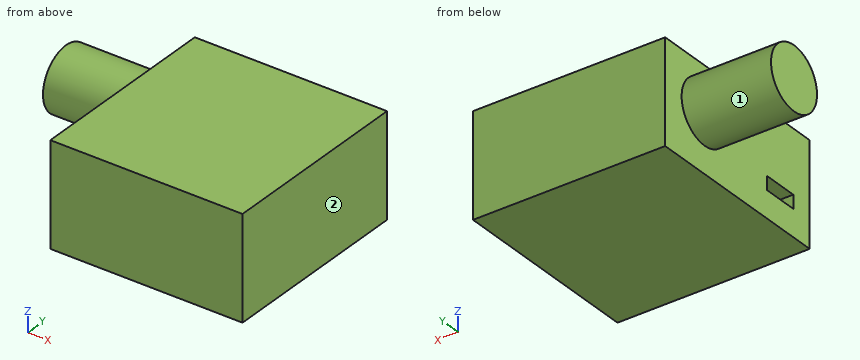
from build123d import *

# Parameters (mm, degrees)
SKETCH009_W             = 44
SKETCH009_H             = 43
PAD006_DEPTH            = 23
SKETCH010_R             = 7
PAD007_DEPTH            = 20
SKETCH011_W             = 8
SKETCH011_H             = 3
POCKET002_DEPTH         = 5
BODY005_PLACEMENT_ANGLE = -90


with BuildPart() as part:
    # Sketch009 → Pad006 (new body)
    with BuildSketch(Plane.XY):
        with Locations((22, 21.5)):
            Rectangle(SKETCH009_W, SKETCH009_H)
    extrude(amount=PAD006_DEPTH)

    # Sketch010 (on Face1 of Pad006) → Pad007 (join)
    with BuildSketch(Plane.XZ):
        with Locations((12, 13)):
            Circle(SKETCH010_R)
    extrude(amount=PAD007_DEPTH)

    # Sketch011 (on Face3 of Pad007) → Pocket002 (cut)
    with BuildSketch(Plane.XZ):
        with Locations((35, 7.5)):
            Rectangle(SKETCH011_W, SKETCH011_H)
    extrude(amount=-POCKET002_DEPTH, mode=Mode.SUBTRACT)


with BuildPart() as part_1:
    # Body005 placement: moved
    add(part.part.moved(Location((1, 248, -23.2))).rotate(Axis((1, 248, -23.2), (0, 0, 1)), BODY005_PLACEMENT_ANGLE))


solid = part_1.part
Build history of the part. All positions in model axes, mm. Face numbers are marked on the shaded views. A direction names the side the tool comes from. Coordinates: 2 decimals unless noted, no trailing zeros. Order: outer loops, then holes, each group sorted by start corner. A loop starts at its lowest first (then second) coordinate and runs counter-clockwise, first axis right, second up. Notation, with made-up numbers: M 7.25,74 L 31.25,74 A21 ccw 31.25,93 Z; hole C -6.5,-27 d4. An arc over 180 degrees is marked long. One line per question, with ' | ' between items. Start each with the question number.
Q1. Saw through at A-A (z = -10.2). List the corners of the cut face in (x, y).
Q2. Probe L1, parallel to X at y = 216.5, z = -5.75; L2, parallel to Y at x = -9, z = -16.5; L3, parallel to Y at x = -7, z = -6. List the from-to ranges inside material, lowest first. Write a range as from..to.
Q3. Saw through at C-C (y = 222). List the corners of the cut face in (x, z).
Q4. Flat gauge pins, fed straight in: pin 1 Ø1.5 at (y, z) = (221.5, -21) entering from -X; pin 2 Ø1 at (x, y) = (-4.5, 235.5) entering from +Z; pin 3 Ø5 at (x, y) = (-11.5, 228) entering from +Z. Where does each tip first touch, or does it go through?
Q5. Saw through at B-B (y = 236). List the corners of the cut face in (x, z), then the cut area to 3 significant figures.
Q6. 3-axis set-ups, long thin cutter, end or side, ignore diameter. For the marked faces 1 and 2: which of +Z, -Z, +X, -X, +Y, -Y reach the whole face in a straight line?
Check values:
1) outline: M -19,229 L 1,229 L 1,204 L 44,204 L 44,248 L 1,248 L 1,243 L -19,243 Z
2) L1: x = 1..44 | L2: y = 232.95..239.05 | L3: y = 230.4..241.6
3) outline: M 1,-23.2 L 44,-23.2 L 44,-0.2 L 1,-0.2 Z
4) pin 1: stops at x = 1 | pin 2: stops at z = -3.2 | pin 3: stops at z = -5.87
5) outline: M -19,-17.2 L 1,-17.2 L 1,-23.2 L 44,-23.2 L 44,-0.2 L 1,-0.2 L 1,-3.2 L -19,-3.2 Z | area: 1,270 mm2
6) face 1: -X | face 2: +Z, -Z, +X, +Y, -Y
